from build123d import *

# Parameters (mm, degrees)
EXTRUDE_1_DEPTH                  = 1
SM_EDGE_FLANGE_1_STRIP_W         = 6
SM_EDGE_FLANGE_1_STRIP_H         = 1
SM_EDGE_FLANGE_1_STRIP_CUT_DEPTH = 410.56637881
SM_EDGE_FLANGE_1_DEPTH           = 410.56637881
CUT_EXTRUDE_1_REACH              = 385.463
SKETCH_12_R                      = 2.5
CUT_EXTRUDE_2_REACH              = 614.164
SKETCH_13_R                      = 2.5


# Sheet-metal steps are written as plain solids
with BuildPart() as part:
    # Sketch 1 → Бобышка-Вытянуть1 (new body)
    with BuildSketch(Plane(origin=(0, 0, 0), x_dir=(0, 0, -1), z_dir=(1, 0, 0))):
        Polygon((223, -275.5), (223, -131.5), (262, -92.5), (262, 76.5), (148.56637881, 238.5), (148.56637881, 275.5), (-262, 275.5), (-262, -275.5), align=None)
    extrude(amount=EXTRUDE_1_DEPTH)

    # Ребро-кромка1 strip (across the edge) → Ребро-кромка1 strip cut (cut)
    with BuildSketch(Plane(origin=(0, 275.5, 262), x_dir=(0, -1, 0), z_dir=(0, 0, -1))):
        with Locations((-1, -0.5)):
            Rectangle(SM_EDGE_FLANGE_1_STRIP_W, SM_EDGE_FLANGE_1_STRIP_H)
    extrude(amount=SM_EDGE_FLANGE_1_STRIP_CUT_DEPTH, mode=Mode.SUBTRACT)

    # Ребро-кромка1 section (across the edge) → Ребро-кромка1 (add)
    with BuildSketch(Plane(origin=(0, 275.5, 262), x_dir=(0, -1, 0), z_dir=(0, 0, -1))):
        with BuildLine():
            Line((0, 1), (0, 50))
            Line((0, 50), (1, 50))
            Line((1, 50), (1, 1))
            ThreePointArc((1, 1), (1.292893219, 0.292893219), (2, 0))
            Line((2, 0), (2, -1))
            ThreePointArc((2, -1), (0.585786438, -0.414213562), (0, 1))
        make_face()
    extrude(amount=SM_EDGE_FLANGE_1_DEPTH)

    # Эскиз12 → Вырез-Вытянуть1 (cut, up to next)
    with BuildSketch(Plane.ZY, mode=Mode.PRIVATE) as cut_extrude_1_sk1:
        with Locations((254, 133.5)):
            Circle(SKETCH_12_R)
    cut_extrude_1_tool1 = extrude(cut_extrude_1_sk1.sketch, amount=-CUT_EXTRUDE_1_REACH, mode=Mode.PRIVATE) & part.part
    # Эскиз12 → Вырез-Вытянуть1 (cut, up to next)
    with BuildSketch(Plane.ZY, mode=Mode.PRIVATE) as cut_extrude_1_sk2:
        with Locations((254, 13.5)):
            Circle(SKETCH_12_R)
    cut_extrude_1_tool2 = extrude(cut_extrude_1_sk2.sketch, amount=-CUT_EXTRUDE_1_REACH, mode=Mode.PRIVATE) & part.part
    # Эскиз12 → Вырез-Вытянуть1 (cut, up to next)
    with BuildSketch(Plane.ZY, mode=Mode.PRIVATE) as cut_extrude_1_sk3:
        with Locations((254, -106.5)):
            Circle(SKETCH_12_R)
    cut_extrude_1_tool3 = extrude(cut_extrude_1_sk3.sketch, amount=-CUT_EXTRUDE_1_REACH, mode=Mode.PRIVATE) & part.part
    # Эскиз12 → Вырез-Вытянуть1 (cut, up to next)
    with BuildSketch(Plane.ZY, mode=Mode.PRIVATE) as cut_extrude_1_sk4:
        with Locations((254, -226.5)):
            Circle(SKETCH_12_R)
    cut_extrude_1_tool4 = extrude(cut_extrude_1_sk4.sketch, amount=-CUT_EXTRUDE_1_REACH, mode=Mode.PRIVATE) & part.part
    # Эскиз12 → Вырез-Вытянуть1 (cut, up to next)
    with BuildSketch(Plane.ZY, mode=Mode.PRIVATE) as cut_extrude_1_sk5:
        with Locations((199.5, -267.5)):
            Circle(SKETCH_12_R)
    cut_extrude_1_tool5 = extrude(cut_extrude_1_sk5.sketch, amount=-CUT_EXTRUDE_1_REACH, mode=Mode.PRIVATE) & part.part
    # Эскиз12 → Вырез-Вытянуть1 (cut, up to next)
    with BuildSketch(Plane.ZY, mode=Mode.PRIVATE) as cut_extrude_1_sk6:
        with Locations((79.5, -267.5)):
            Circle(SKETCH_12_R)
    cut_extrude_1_tool6 = extrude(cut_extrude_1_sk6.sketch, amount=-CUT_EXTRUDE_1_REACH, mode=Mode.PRIVATE) & part.part
    # Эскиз12 → Вырез-Вытянуть1 (cut, up to next)
    with BuildSketch(Plane.ZY, mode=Mode.PRIVATE) as cut_extrude_1_sk7:
        with Locations((-40.5, -267.5)):
            Circle(SKETCH_12_R)
    cut_extrude_1_tool7 = extrude(cut_extrude_1_sk7.sketch, amount=-CUT_EXTRUDE_1_REACH, mode=Mode.PRIVATE) & part.part
    # Эскиз12 → Вырез-Вытянуть1 (cut, up to next)
    with BuildSketch(Plane.ZY, mode=Mode.PRIVATE) as cut_extrude_1_sk8:
        with Locations((-160.5, -267.5)):
            Circle(SKETCH_12_R)
    cut_extrude_1_tool8 = extrude(cut_extrude_1_sk8.sketch, amount=-CUT_EXTRUDE_1_REACH, mode=Mode.PRIVATE) & part.part
    # Эскиз12 → Вырез-Вытянуть1 (cut, up to next)
    with BuildSketch(Plane.ZY, mode=Mode.PRIVATE) as cut_extrude_1_sk9:
        with Locations((-215, -226.5)):
            Circle(SKETCH_12_R)
    cut_extrude_1_tool9 = extrude(cut_extrude_1_sk9.sketch, amount=-CUT_EXTRUDE_1_REACH, mode=Mode.PRIVATE) & part.part
    # Эскиз12 → Вырез-Вытянуть1 (cut, up to next)
    with BuildSketch(Plane.ZY, mode=Mode.PRIVATE) as cut_extrude_1_sk10:
        with Locations((-236.686291501, -106.5)):
            Circle(SKETCH_12_R)
    cut_extrude_1_tool10 = extrude(cut_extrude_1_sk10.sketch, amount=-CUT_EXTRUDE_1_REACH, mode=Mode.PRIVATE) & part.part
    # Эскиз12 → Вырез-Вытянуть1 (cut, up to next)
    with BuildSketch(Plane.ZY, mode=Mode.PRIVATE) as cut_extrude_1_sk11:
        with Locations((-253.890872965, 13.5)):
            Circle(SKETCH_12_R)
    cut_extrude_1_tool11 = extrude(cut_extrude_1_sk11.sketch, amount=-CUT_EXTRUDE_1_REACH, mode=Mode.PRIVATE) & part.part
    # Эскиз12 → Вырез-Вытянуть1 (cut, up to next)
    with BuildSketch(Plane.ZY, mode=Mode.PRIVATE) as cut_extrude_1_sk12:
        with Locations((-212.321973612, 133.5)):
            Circle(SKETCH_12_R)
    cut_extrude_1_tool12 = extrude(cut_extrude_1_sk12.sketch, amount=-CUT_EXTRUDE_1_REACH, mode=Mode.PRIVATE) & part.part
    add(cut_extrude_1_tool1.solids().sort_by_distance((0, 133.5, 254))[0], mode=Mode.SUBTRACT)
    add(cut_extrude_1_tool2.solids().sort_by_distance((0, 13.5, 254))[0], mode=Mode.SUBTRACT)
    add(cut_extrude_1_tool3.solids().sort_by_distance((0, -106.5, 254))[0], mode=Mode.SUBTRACT)
    add(cut_extrude_1_tool4.solids().sort_by_distance((0, -226.5, 254))[0], mode=Mode.SUBTRACT)
    add(cut_extrude_1_tool5.solids().sort_by_distance((0, -267.5, 199.5))[0], mode=Mode.SUBTRACT)
    add(cut_extrude_1_tool6.solids().sort_by_distance((0, -267.5, 79.5))[0], mode=Mode.SUBTRACT)
    add(cut_extrude_1_tool7.solids().sort_by_distance((0, -267.5, -40.5))[0], mode=Mode.SUBTRACT)
    add(cut_extrude_1_tool8.solids().sort_by_distance((0, -267.5, -160.5))[0], mode=Mode.SUBTRACT)
    add(cut_extrude_1_tool9.solids().sort_by_distance((0, -226.5, -215))[0], mode=Mode.SUBTRACT)
    add(cut_extrude_1_tool10.solids().sort_by_distance((0, -106.5, -236.686292))[0], mode=Mode.SUBTRACT)
    add(cut_extrude_1_tool11.solids().sort_by_distance((0, 13.5, -253.890873))[0], mode=Mode.SUBTRACT)
    add(cut_extrude_1_tool12.solids().sort_by_distance((0, 133.5, -212.321974))[0], mode=Mode.SUBTRACT)

    # Эскиз13 → Вырез-Вытянуть2 (cut, up to next)
    with BuildSketch(Plane(origin=(0, 275.5, 0), x_dir=(1, 0, 0), z_dir=(0, 1, 0)), mode=Mode.PRIVATE) as cut_extrude_2_sk1:
        with Locations(Location((-43, -196.716810595, 0), (0, 0, 180))):
            Circle(SKETCH_13_R)
    cut_extrude_2_tool1 = extrude(cut_extrude_2_sk1.sketch, amount=-CUT_EXTRUDE_2_REACH, mode=Mode.PRIVATE) & part.part
    # Эскиз13 → Вырез-Вытянуть2 (cut, up to next)
    with BuildSketch(Plane(origin=(0, 275.5, 0), x_dir=(1, 0, 0), z_dir=(0, 1, 0)), mode=Mode.PRIVATE) as cut_extrude_2_sk2:
        with Locations(Location((-43, -56.716810595, 0), (0, 0, 180))):
            Circle(SKETCH_13_R)
    cut_extrude_2_tool2 = extrude(cut_extrude_2_sk2.sketch, amount=-CUT_EXTRUDE_2_REACH, mode=Mode.PRIVATE) & part.part
    # Эскиз13 → Вырез-Вытянуть2 (cut, up to next)
    with BuildSketch(Plane(origin=(0, 275.5, 0), x_dir=(1, 0, 0), z_dir=(0, 1, 0)), mode=Mode.PRIVATE) as cut_extrude_2_sk3:
        with Locations(Location((-43, 83.283189405, 0), (0, 0, 180))):
            Circle(SKETCH_13_R)
    cut_extrude_2_tool3 = extrude(cut_extrude_2_sk3.sketch, amount=-CUT_EXTRUDE_2_REACH, mode=Mode.PRIVATE) & part.part
    add(cut_extrude_2_tool1.solids().sort_by_distance((-43, 275.5, 196.716811))[0], mode=Mode.SUBTRACT)
    add(cut_extrude_2_tool2.solids().sort_by_distance((-43, 275.5, 56.716811))[0], mode=Mode.SUBTRACT)
    add(cut_extrude_2_tool3.solids().sort_by_distance((-43, 275.5, -83.283189))[0], mode=Mode.SUBTRACT)


solid = part.part
The model under review builds one solid part; all positions refer to its coordinate system, in mm. A direction names the side the tool comes from. Round coordinates to 2 decimals unless told otherwise and drop trailing zeros. Loops run counter-clockwise (first coordinate to the right, second up) from the corner with the lowest first, then second, coordinate; pieces in that order, holes last. Notation, with made-up numbers: (58, 40.5) -> (68, 40.5) arc R21 ccw to (68, 74.5) -> close; hole circle Ø5 at (60.25, 29.25). An arc over 180 degrees is marked (long way). One line per question, with ' | ' between items. Start each with the question number.
Item 1: Machinability: for faces 1 (the face through (0, 3, 4)), 2 (the face through (1, 3, 4)), which of the approach directions +Z, -Z, +X, -X, +Y, -Y give a long, thin tool a straight path to every point of the face, cutting with its end or side? Answer none if there is none.
Item 2: Wall thickness on line 1 along Z through (x, y) = (-43, 275.1); line 2 along Z through (x, y) = (0.4, -226.5); line 3 along Y through (x, z) = (0.3, 254): over which ranges is each line inside the solid? List them lowest first. Write a range as [from, to].
Item 3: Add section C-C, the plane x = -8. Write out the cut boundary in (y, z), then the cut area to 3 significant figures.
Item 4: Add section B-B, the plane y = -24. Write out the cut boundary in (x, z).
Item 5: For pin 1 (6.5 mm diameter, centred on y = 133.5, z = 254, fed in from -X); pin 2 (8 mm diameter, centred on x = -43, z = -83.28, fed in from -Y); pin 3 (1.1 mm diameter, centred on x = 0.5, y = -173, fed in from -Z), all flat-tipped, find the tip position at first contact; note any pin that passes through.
Item 6: Add section A-A, the plane z = 95. Write out the cut boundary in (x, y), then the cut area to 3 significant figures.
Return value:
1) face 1: +Z, -Z, -X, -Y | face 2: +Z, -Z, +X, +Y, -Y
2) line 1: z = [-148.57, -85.78], [-80.78, 54.22], [59.22, 194.22], [199.22, 262] | line 2: z = [-223, -217.5], [-212.5, 251.5], [256.5, 262] | line 3: y = [-275.5, -229], [-224, -109], [-104, 11], [16, 131], [136, 275.02]
3) outline: (274.5, -148.57) -> (275.5, -148.57) -> (275.5, 262) -> (274.5, 262) -> close | area: 411 mm2
4) outline: (0, -262) -> (1, -262) -> (1, 262) -> (0, 262) -> close
5) pin 1: stops at x = 0 | pin 2: stops at y = 274.5 | pin 3: stops at z = -223
6) outline: (-50, 274.5) -> (-1, 274.5) arc R1 cw to (0, 273.5) -> (0, -275.5) -> (1, -275.5) -> (1, 273.5) arc R2 ccw to (-1, 275.5) -> (-50, 275.5) -> close | area: 600 mm2
